```python
from build123d import *

# Parameters (mm, degrees)
ESQUISSE1_W             = 42
ESQUISSE1_H             = 42
BOSS_EXTRU_6_DEPTH      = 12
ESQUISSE9_W             = 42
ESQUISSE9_H             = 13
BOSS_EXTRU_7_DEPTH      = 40
ESQUISSE10_W            = 42
ESQUISSE10_H            = 42
BOSS_EXTRU_8_DEPTH      = 13
ESQUISSE12_R            = 4.5
ENL_V_MAT_EXTRU_3_DEPTH = 72.463277283
ESQUISSE13_W            = 42
ESQUISSE13_H            = 5
ENL_V_MAT_EXTRU_4_DEPTH = 72.463277283
ESQUISSE15_W            = 4
ESQUISSE15_H            = 32
ENL_V_MAT_EXTRU_5_DEPTH = 71.809603868


with BuildPart() as part:
    # Esquisse1 → Boss.-Extru.6 (new body)
    with BuildSketch(Plane(origin=(0, 0, 0), x_dir=(1, 0, 0), z_dir=(0, 1, 0))):
        Rectangle(ESQUISSE1_W, ESQUISSE1_H)
    extrude(amount=BOSS_EXTRU_6_DEPTH)

    # Esquisse9 → Boss.-Extru.7 (add)
    with BuildSketch(Plane.XZ):
        with Locations((0, -14.5)):
            Rectangle(ESQUISSE9_W, ESQUISSE9_H)
        with Locations((0, 14.5)):
            Rectangle(ESQUISSE9_W, ESQUISSE9_H)
    extrude(amount=BOSS_EXTRU_7_DEPTH)

    # Esquisse10 → Boss.-Extru.8 (add)
    with BuildSketch(Plane.XZ.offset(40)):
        Rectangle(ESQUISSE10_W, ESQUISSE10_H)
    extrude(amount=BOSS_EXTRU_8_DEPTH)

    # Esquisse12 → Enlèv. mat.-Extru.3 (cut, through all)
    with BuildSketch(Plane(origin=(0, 12, 0), x_dir=(1, 0, 0), z_dir=(0, 1, 0))):
        with Locations(Location((0, 0, 0), (0, 0, 270))):
            Circle(ESQUISSE12_R)
    extrude(amount=-ENL_V_MAT_EXTRU_3_DEPTH, mode=Mode.SUBTRACT)

    # Esquisse13 → Enlèv. mat.-Extru.4 (cut, through all)
    with BuildSketch(Plane(origin=(0, 12, 0), x_dir=(1, 0, 0), z_dir=(0, 1, 0))):
        with Locations((0, 18.5)):
            Rectangle(ESQUISSE13_W, ESQUISSE13_H)
    extrude(amount=-ENL_V_MAT_EXTRU_4_DEPTH, mode=Mode.SUBTRACT)

    # Esquisse15 → Enlèv. mat.-Extru.5 (cut, through all)
    with BuildSketch(Plane(origin=(21, 0, 0), x_dir=(0, 0, -1), z_dir=(1, 0, 0))):
        with Locations((14, -20.5)):
            Rectangle(ESQUISSE15_W, ESQUISSE15_H)
    extrude(amount=-ENL_V_MAT_EXTRU_5_DEPTH, mode=Mode.SUBTRACT)


solid = part.part
```
CAD build for the part. Positions are in the model's coordinates, mm. A direction names the side the tool comes from. Round coordinates to 2 decimals unless told otherwise and drop trailing zeros. Write each loop counter-clockwise with the first axis right and the second up, starting at its lowest first coordinate (ties: lowest second). Pieces come first, ordered by that corner, then holes. Notation, with made-up numbers: (31, 78.5) - (79, 78.5) arc R31 cw to (79, 113.5) - close; hole circle Ø1 at (45, 43). An arc over 180 degrees is marked (long way). Return JSON: item names as keys, results as strings. Group by question number.
Item 1: Probe probe 1 along Y at (x, z) = (4, -13); probe 2 along Z at (x, y) = (-2, -28.5); probe 3 along Y at (x, z) = (14, 2). List the from-to ranges inside material, lowest first.
Item 2: Flat gauge pins, fed straight in: pin 1 Ø20 at (x, y) = (-2.5, -19) entering from -Z; pin 2 Ø8 at (x, z) = (0, 0) entering from +Y. Where does each tip first touch, or does it go through?
Item 3: Band-saw the part on D-D on x = 15.5. List the corners of the cut face in (y, z), plus the area to 3 significant figures.
Item 4: 3-axis set-ups, long thin cutter, end or side, ignore diameter. For faces 1 (the face through (0, -4.5, -14)), 2 (the face through (-5, 0, 0)), 3 (the face through (1.352, 6.084, 4.292)): which of +Z, -Z, +X, -X, +Y, -Y reach the whole face in a straight line?
Item 5: Band-saw the part on A-A on z = 5.5. List the corners of the cut face in (x, y).
Item 6: Mould opens along Y. For faces 4 (the face through (0, -20, 21)), 5 (the face through (0, -53, 7)), 6 (the face through (0, -36.5, -14)) say: +Y half, -Y half, draft (parallel to the pull), parting line (faces both ways), or undercut.
Item 7: Band-saw the part on B-B on x = 0. List the corners of the cut face in (y, z).
Item 8: Band-saw the part on C-C on y = 2. List the corners of the cut face in (x, z), plus the area to 3 significant figures.
Resolved:
{
 "1": {"probe 1": "y = -53 to -36.5, -4.5 to 12", "probe 2": "z = -12 to -8, 8 to 21", "probe 3": "y = -53 to -40, 0 to 12"},
 "2": {"pin 1": "stops at z = -12", "pin 2": "passes through"},
 "3": {"outline": "(-53, -16) - (-36.5, -16) - (-36.5, -12) - (-4.5, -12) - (-4.5, -16) - (12, -16) - (12, 21) - (-53, 21) - close; hole (-40, -8) - (0, -8) - (0, 8) - (-40, 8) - close", "area": "1,640 mm²"},
 "4": {"face 1": "-Z, +X, -X", "face 2": "+X, -X", "face 3": "+Y, -Y"},
 "5": {"outline": "(-21, -53) - (21, -53) - (21, -40) - (-21, -40) - close; (-21, 0) - (21, 0) - (21, 12) - (-21, 12) - close"},
 "6": {"face 4": "draft", "face 5": "-Y half", "face 6": "undercut"},
 "7": {"outline": "(-53, -16) - (-36.5, -16) - (-36.5, -12) - (-4.5, -12) - (-4.5, -16) - (12, -16) - (12, -4.5) - (0, -4.5) - (0, -8) - (-40, -8) - (-40, -4.5) - (-53, -4.5) - close; (-53, 4.5) - (-40, 4.5) - (-40, 8) - (0, 8) - (0, 4.5) - (12, 4.5) - (12, 21) - (-53, 21) - close"},
 "8": {"outline": "(-21, -16) - (21, -16) - (21, 21) - (-21, 21) - close; hole circle Ø9 at (0, 0)", "area": "1,490 mm²"}
}
